Geometry check sheet. Reference: the model listing, model coordinates, mm. Face numbers are marked on the shaded views. A direction names the side the tool comes from. Coordinates: 2 decimals unless noted, no trailing zeros. Write each loop counter-clockwise with the first axis right and the second up, starting at its lowest first coordinate (ties: lowest second). Pieces come first, ordered by that corner, then holes. Notation, with made-up numbers: (39.25, 3) -> (67.25, 3) arc R12 ccw to (67.25, 17) -> close; hole circle Ø2 at (-10, 29.5). An arc over 180 degrees is marked (long way). One line per question, with ' | ' between items.
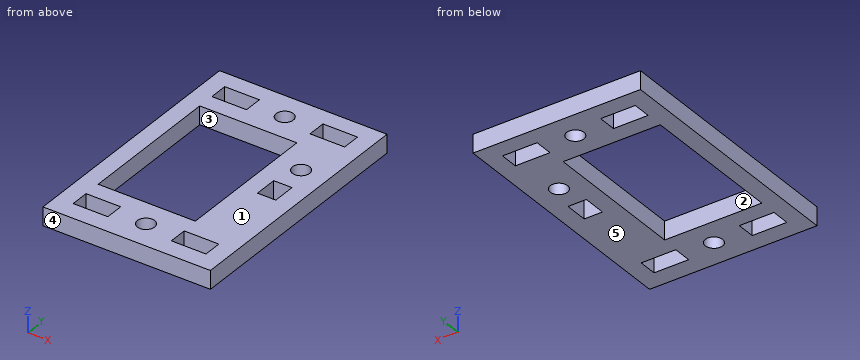
from build123d import *

# Parameters (mm, degrees)
F0_W     = 29
F0_H     = 43.5875
F0_W_2   = 6
F0_H_2   = 3.175
F0_R     = 1.5
F0_W_3   = 16.825
F0_H_3   = 25.0625
F0_W_4   = 3.175
F0_H_4   = 4
F1_DEPTH = 3.175


# Not quite as in the source:
# - a length typed as a fraction of an inch, garbled in the dataset ("3 / 203.2 mm" for 3/8 in), is restored


with BuildPart() as f1:
    # F0 (on Top) → F1 (new body)
    with BuildSketch(Plane.XY):
        with Locations((-29.1205597607, 9.4016398251)):
            Rectangle(F0_W, F0_H)
        with Locations((-37.6205597607, -7.6296101749)):
            Rectangle(F0_W_2, F0_H_2, mode=Mode.SUBTRACT)
        with Locations((-29.1205597607, -7.6296101749)):
            Circle(F0_R, mode=Mode.SUBTRACT)
        with Locations((-20.6205597607, -7.6296101749)):
            Rectangle(F0_W_2, F0_H_2, mode=Mode.SUBTRACT)
        with Locations((-32.2080597607, 9.4891398251)):
            Rectangle(F0_W_3, F0_H_3, mode=Mode.SUBTRACT)
        with Locations((-37.6205597607, 26.6078898251)):
            Rectangle(F0_W_2, F0_H_2, mode=Mode.SUBTRACT)
        with Locations((-19.2080597607, 10.0203898251)):
            Rectangle(F0_W_4, F0_H_4, mode=Mode.SUBTRACT)
        with Locations((-19.2080597607, 16.5203898251)):
            Circle(F0_R, mode=Mode.SUBTRACT)
        with Locations((-29.1205597607, 26.6078898251)):
            Circle(F0_R, mode=Mode.SUBTRACT)
        with Locations((-20.6205597607, 26.6078898251)):
            Rectangle(F0_W_2, F0_H_2, mode=Mode.SUBTRACT)
    extrude(amount=F1_DEPTH)


solid = f1.part
1. Go/stop test with a flat-tipped pin: P1, Ø2.5, axis at x = -29.12, y = 26.61, coming from the -Z side. Record where the tip stops, or that it passes through.
Worked answers:
P1: through
2. Cross-section at A-A on y = -1.5. Record the boundary of the cut face in (x, z) (3 decimals), and give its area (3 significant figures).
Worked answers:
outline: (-43.621, 0) -> (-40.621, 0) -> (-40.621, 3.175) -> (-43.621, 3.175) -> close; (-23.796, 0) -> (-14.621, 0) -> (-14.621, 3.175) -> (-23.796, 3.175) -> close | area: 38.7 mm²
3. Cross-section at D-D on z = 2.2. Give the number of separate pieces and of enclosed holes in the cut face, and give its area (3 significant figures).
Worked answers:
separate pieces: 1 | enclosed holes: 9 | area: 732 mm²
4. Mould release check, pull along Y, two halves, no side actions. Record for the marked faces 3, 4 and 5: released by +Y, released by -Y, zero draft, split by the parting line, or undercut.
Worked answers:
face 3: undercut | face 4: released by -Y | face 5: zero draft
5. Material ranges on line 1 (Y direction, x = -22, z = 0.2); line 2 (Y direction, x = -37.5, z = 1.4); line 3 (X direction, y = 11, z = 0.9), recorded low to high. Write a range as from..to.
Worked answers:
line 1: -12.39..-9.22, -6.04..25.02, 28.2..31.2 | line 2: -12.39..-9.22, -6.04..-3.04, 22.02..25.02, 28.2..31.2 | line 3: -43.62..-40.62, -23.8..-20.8, -17.62..-14.62
6. Cross-section at B-B on y = 9. Record the boundary of the cut face in (x, z) (3 decimals).
Worked answers:
outline: (-43.621, 0) -> (-40.621, 0) -> (-40.621, 3.175) -> (-43.621, 3.175) -> close; (-23.796, 0) -> (-20.796, 0) -> (-20.796, 3.175) -> (-23.796, 3.175) -> close; (-17.621, 0) -> (-14.621, 0) -> (-14.621, 3.175) -> (-17.621, 3.175) -> close
7. Tool access check on the marked faces 1 and 2. Record the directions out of +Z, -Z, +X, -X, +Y, -Y that give a thin tool (end or side, any length) a straight path to the whole face; none if there is none.
Worked answers:
face 1: +Z, +X, -X, +Y, -Y | face 2: +Z, -Z
8. Cross-section at C-C on x = -39. Record the boundary of the cut face in (y, z) (3 decimals).
Worked answers:
outline: (-12.392, 0) -> (-9.217, 0) -> (-9.217, 3.175) -> (-12.392, 3.175) -> close; (-6.042, 0) -> (-3.042, 0) -> (-3.042, 3.175) -> (-6.042, 3.175) -> close; (22.02, 0) -> (25.02, 0) -> (25.02, 3.175) -> (22.02, 3.175) -> close; (28.195, 0) -> (31.195, 0) -> (31.195, 3.175) -> (28.195, 3.175) -> close
